from build123d import *

# Parameters (mm, degrees)
BOSS_EXTRUDE1_DEPTH = 45
SKETCH4_W           = 12
SKETCH4_H           = 10
SKETCH4_R           = 2.2
BOSS_EXTRUDE2_DEPTH = 3
FILLET1_R           = 4
FILLET2_R           = 2
FILLET3_R           = 2


with BuildPart() as part:
    # Sketch3 → Boss-Extrude1 (new body)
    with BuildSketch(Plane(origin=(0, 0, 0), x_dir=(1, 0, 0), z_dir=(0, 1, 0))):
        with BuildLine():
            Line((-8, 24), (-29, 24))
            ThreePointArc((-29, 24), (-31.121320344, 23.121320344), (-32, 21))
            Line((-32, 21), (-32, -21))
            ThreePointArc((-32, -21), (-31.121320344, -23.121320344), (-29, -24))
            Line((-29, -24), (-8, -24))
            Line((-8, -24), (-8, -27))
            Line((-8, -27), (-29, -27))
            ThreePointArc((-29, -27), (-33.242640687, -25.242640687), (-35, -21))
            Line((-35, -21), (-35, 21))
            ThreePointArc((-35, 21), (-33.242640687, 25.242640687), (-29, 27))
            Line((-29, 27), (-8, 27))
            Line((-8, 27), (-8, 24))
        make_face()
    extrude(amount=BOSS_EXTRUDE1_DEPTH)

    # Sketch4 → Boss-Extrude2 (add)
    # profile 1 of 2: a face of its own
    with BuildSketch(Plane(origin=(0, 45, 0), x_dir=(1, 0, 0), z_dir=(0, 1, 0))):
        with Locations((-41, 12)):
            Rectangle(SKETCH4_W, SKETCH4_H)
        with Locations(Location((-42, 12, 0), (0, 0, 270))):
            Circle(SKETCH4_R, mode=Mode.SUBTRACT)
    # profile 2 of 2: a face of its own
    with BuildSketch(Plane(origin=(0, 45, 0), x_dir=(1, 0, 0), z_dir=(0, 1, 0))):
        with Locations((-41, -12)):
            Rectangle(SKETCH4_W, SKETCH4_H)
        with Locations(Location((-42, -12, 0), (0, 0, 270))):
            Circle(SKETCH4_R, mode=Mode.SUBTRACT)
    extrude(amount=-BOSS_EXTRUDE2_DEPTH)

    # Fillet1
    fillet1_edges = [part.edges().sort_by_distance(p)[0] for p in [
        (-35, 43.5, -17),
        (-35, 43.5, -7),
        (-35, 43.5, 7),
        (-35, 43.5, 17),
    ]]
    fillet(fillet1_edges, radius=FILLET1_R - 0.0001)  # a hair under: the kernel refuses the full size

    # Fillet2
    fillet2_edges = [part.edges().sort_by_distance(p)[0] for p in [
        (-35, 42, -12),
        (-35, 42, 12),
    ]]
    fillet(fillet2_edges, radius=FILLET2_R)

    # Fillet3
    fillet3_edges = [part.edges().sort_by_distance(p)[0] for p in [
        (-47, 43.5, -7),
        (-47, 43.5, -17),
        (-47, 43.5, 17),
        (-47, 43.5, 7),
    ]]
    fillet(fillet3_edges, radius=FILLET3_R)


solid = part.part
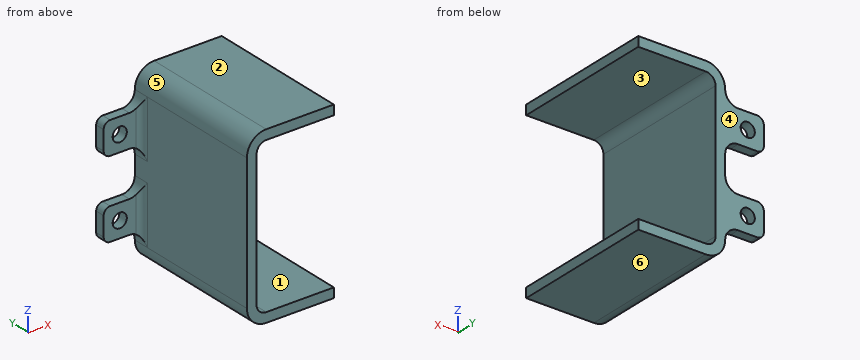
Input: part model. Units: mm. Frame: model coordinates. Face numbers are marked on the shaded views. A direction names the side the tool comes from. Round coordinates to 2 decimals unless told otherwise and drop trailing zeros. Order: outer loops, then holes, each group sorted by start corner. A loop starts at its lowest first (then second) coordinate and runs counter-clockwise, first axis right, second up.
1. Material intervals for line 1 (Z direction, x = -11.5, y = 6); line 2 (X direction, y = 43, z = 12); line 3 (Y direction, x = -39, z = 12), sorted ascending.
The answers:
line 1: z = -27 to -24, 24 to 27
line 2: x = -47 to -44.2, -39.8 to -32
line 3: y = 42 to 45
2. Cut plane B-B, the plane z = -12. Output: boundary loops of the cut face in (x, y), then the cut area to 3 significant figures.
The answers:
outline: (-47, 42) - (-44.2, 42) - (-44.2, 45) - (-47, 45) - close; (-39.8, 42) - (-37, 42) arc R2 cw to (-35, 40) - (-35, 0) - (-32, 0) - (-32, 45) - (-39.8, 45) - close
area: 159 mm2
3. Set-up query: the marked faces 1 and 2. Return all of +Z, -Z, +X, -X, +Y, -Y with unobstructed straight access to the full face (end or side cutting, diameter ignored); none if empty.
The answers:
face 1: +X, +Y, -Y
face 2: +Z, +X, -X, +Y, -Y
4. Cut plane A-A, the plane x = -19.5. Output: boundary loops of the cut face in (y, z), then the cut area to 3 significant figures.
The answers:
outline: (0, -27) - (45, -27) - (45, -24) - (0, -24) - close; (0, 24) - (45, 24) - (45, 27) - (0, 27) - close
area: 270 mm2
5. Cut plane C-C, the plane x = -42. Output: boundary loops of the cut face in (y, z), then the cut area to 3 significant figures.
The answers:
outline: (42, -17) - (45, -17) - (45, -14.2) - (42, -14.2) - close; (42, -9.8) - (45, -9.8) - (45, -7) - (42, -7) - close; (42, 7) - (45, 7) - (45, 9.8) - (42, 9.8) - close; (42, 14.2) - (45, 14.2) - (45, 17) - (42, 17) - close
area: 33.6 mm2
6. Pin query (flat end, axial travel): P1, Ø3.5, axis at x = -42, y = 44, coming from the +Z side; P2, Ø12.5, axis at y = 30.5, z = -4.5, coming from the -X side; P3, Ø6, axis at x = -41.5, z = -13.5, coming from the -Y side. Return the tip coordinate at first contact, or that it passes through.
The answers:
P1: stops at z = 17
P2: stops at x = -35
P3: stops at y = 42
7. Mould query, pull axis Z, two halves, no side actions, for the marked faces 3, 4, 5 and 6. Classes: released by +Z, released by -Z, zero draft, split by the parting line, or undercut.
The answers:
face 3: undercut
face 4: zero draft
face 5: released by +Z
face 6: released by -Z
8. Cut plane D-D, the plane y = 33. Output: boundary loops of the cut face in (x, z), then the cut area to 3 significant figures.
The answers:
outline: (-35, -21) arc R6 ccw to (-29, -27) - (-8, -27) - (-8, -24) - (-29, -24) arc R3 cw to (-32, -21) - (-32, 21) arc R3 cw to (-29, 24) - (-8, 24) - (-8, 27) - (-29, 27) arc R6 ccw to (-35, 21) - close
area: 294 mm2
